from build123d import *

# Parameters (mm, degrees)
SKETCH_1_R      = 2.15
SKETCH_1_R_2    = 1.65
EXTRUDE_1_DEPTH = 3
FILLET_1_R      = 1


with BuildPart() as part:
    # 草图1 → 凸台-拉伸1 (new body)
    with BuildSketch(Plane.XY):
        Polygon((7.5, 32.5), (17.5, 32.5), (17.5, -2.5), (7.5, -2.5), (7.5, -7.5), (-7.5, -7.5), (-7.5, 32.5), align=None)
        Circle(SKETCH_1_R, mode=Mode.SUBTRACT)
        with Locations((0, 25)):
            Circle(SKETCH_1_R, mode=Mode.SUBTRACT)
        with Locations((12.5, 24.5)):
            Circle(SKETCH_1_R_2, mode=Mode.SUBTRACT)
        with Locations((12.5, 6.5)):
            Circle(SKETCH_1_R_2, mode=Mode.SUBTRACT)
    extrude(amount=EXTRUDE_1_DEPTH)

    # 圆角1
    fillet_1_edges = [part.edges().sort_by_distance(p)[0] for p in [
        (7.5, -7.5, 1.5),
        (-7.5, -7.5, 1.5),
        (-7.5, 32.5, 1.5),
        (17.5, 32.5, 1.5),
        (17.5, -2.5, 1.5),
        (7.5, -2.5, 1.5),
    ]]
    fillet(fillet_1_edges, radius=FILLET_1_R)


solid = part.part
Input: part model. Units: mm. Frame: model coordinates. A direction names the side the tool comes from. Coordinates: 2 decimals unless noted, no trailing zeros. Loops run counter-clockwise (first coordinate to the right, second up) from the corner with the lowest first, then second, coordinate; pieces in that order, holes last.
(1) First-contact query: pin 1 Ø2.5 at (x, y) = (12.5, 6.5) entering from -Z; pin 2 Ø0.9 at (x, z) = (12, 2) entering from -Y. Flat tips, straight axial feed; report the tip coordinate or a pass-through.
(2) Material intervals for probe 1 along Y at (x, z) = (12.5, 1.45); probe 2 along Y at (x, z) = (0, 1.6); probe 3 along Y at (x, z) = (16.25, 0.95), sorted ascending.
(3) Section D-D on x = 0. Return the cut outline in (y, z), then the cut area to 3 significant figures.
(4) Section C-C on z = 2.2. Return the cut outline in (x, y), then the cut area to 3 significant figures.
(5) Section B-B on y = 6.5. Return the cut outline in (x, z), then the cut area to 3 significant figures.
(6) Set-up query: faces 1 (the face through (-7.215, -7.199, 1.521)), 2 (the face through (13, -2.5, 1)). Return all of +Z, -Z, +X, -X, +Y, -Y with unobstructed straight access to the full face (end or side cutting, diameter ignored); none if empty.
(7) Pull-direction query (X, two-part tool) for faces 3 (the face through (5, 13, 3)), 4 (the face through (7.199, -7.215, 1.521)), 5 (the face through (14.024, 5.868, 1.479)); classes: released by +X, released by -X, zero draft, split by the parting line, or undercut.
(8) Section A-A on x = 12.5. Return the cut outline in (y, z).
Data:
1. pin 1: passes through
1. pin 2: stops at y = -2.5
2. probe 1: y = -2.5 to 4.85, 8.15 to 22.85, 26.15 to 32.5
2. probe 2: y = -7.5 to -2.15, 2.15 to 22.85, 27.15 to 32.5
2. probe 3: y = -2.5 to 32.5
3. outline: (-7.5, 0) - (-2.15, 0) - (-2.15, 3) - (-7.5, 3) - close; (2.15, 0) - (22.85, 0) - (22.85, 3) - (2.15, 3) - close; (27.15, 0) - (32.5, 0) - (32.5, 3) - (27.15, 3) - close
3. area: 94.2 mm2
4. outline: (-7.5, -6.5) arc R1 ccw to (-6.5, -7.5) - (6.5, -7.5) arc R1 ccw to (7.5, -6.5) - (7.5, -3.5) arc R1 cw to (8.5, -2.5) - (16.5, -2.5) arc R1 ccw to (17.5, -1.5) - (17.5, 31.5) arc R1 ccw to (16.5, 32.5) - (-6.5, 32.5) arc R1 ccw to (-7.5, 31.5) - close; hole circle Ø4.3 at (0, 0); hole circle Ø4.3 at (0, 25); hole circle Ø3.3 at (12.5, 6.5); hole circle Ø3.3 at (12.5, 24.5)
4. area: 903 mm2
5. outline: (-7.5, 0) - (10.85, 0) - (10.85, 3) - (-7.5, 3) - close; (14.15, 0) - (17.5, 0) - (17.5, 3) - (14.15, 3) - close
5. area: 65.1 mm2
6. face 1: +Z, -Z, -X, -Y
6. face 2: +Z, -Z, +X, -Y
7. face 3: zero draft
7. face 4: released by +X
7. face 5: undercut
8. outline: (-2.5, 0) - (4.85, 0) - (4.85, 3) - (-2.5, 3) - close; (8.15, 0) - (22.85, 0) - (22.85, 3) - (8.15, 3) - close; (26.15, 0) - (32.5, 0) - (32.5, 3) - (26.15, 3) - close
